Here's how the part is built. I have some questions about the finished solid (model axes, mm). A direction names the side the tool comes from. Coordinates: 2 decimals unless noted, no trailing zeros. Write each loop counter-clockwise with the first axis right and the second up, starting at its lowest first coordinate (ties: lowest second). Pieces come first, ordered by that corner, then holes.
```python
from build123d import *

# Parameters (mm, degrees)
SKETCH1_W           = 15
SKETCH1_H           = 100
BOSS_EXTRUDE1_DEPTH = 103
SKETCH2_W           = 15
SKETCH2_H           = 2
BOSS_EXTRUDE2_DEPTH = 15
SKETCH3_W           = 15
SKETCH3_H           = 2
BOSS_EXTRUDE3_DEPTH = 15
SKETCH4_R           = 2.15
CUT_EXTRUDE1_DEPTH  = 15
CHAMFER1_SIZE       = 1


with BuildPart() as part:
    # Sketch1 → Boss-Extrude1 (new body)
    with BuildSketch(Plane(origin=(0, 0, 0), x_dir=(1, 0, 0), z_dir=(0, 1, 0))):
        with Locations((7.5, 50)):
            Rectangle(SKETCH1_W, SKETCH1_H)
    extrude(amount=BOSS_EXTRUDE1_DEPTH)

    # Sketch2 → Boss-Extrude2 (add)
    with BuildSketch(Plane.ZY):
        with Locations((-50, 1)):
            Rectangle(SKETCH2_W, SKETCH2_H)
    extrude(amount=BOSS_EXTRUDE2_DEPTH)

    # Sketch3 → Boss-Extrude3 (add)
    with BuildSketch(Plane(origin=(15, 0, 0), x_dir=(0, 0, -1), z_dir=(1, 0, 0))):
        with Locations((50, 1)):
            Rectangle(SKETCH3_W, SKETCH3_H)
    extrude(amount=BOSS_EXTRUDE3_DEPTH)

    # Sketch4 → Cut-Extrude1 (cut)
    with BuildSketch(Plane(origin=(0, 2, 0), x_dir=(1, 0, 0), z_dir=(0, 1, 0))):
        with Locations(Location((-7.5, 50, 0), (0, 0, 270))):
            Circle(SKETCH4_R)
        with Locations(Location((22.5, 50, 0), (0, 0, 270))):
            Circle(SKETCH4_R)
    extrude(amount=-CUT_EXTRUDE1_DEPTH, mode=Mode.SUBTRACT)

    # Chamfer1
    chamfer1_edges = [part.edges().sort_by_distance(p)[0] for p in [
        (-7.5, 2, -52.15),
        (22.5, 2, -52.15),
    ]]
    chamfer(chamfer1_edges, length=CHAMFER1_SIZE)


solid = part.part
```
1) Imagine slicing it at B-B on x = -7.5. Please give me the cut outline in (y, z), then the cut area to 3 significant figures.
Values follow:
outline: (0, -57.5) - (2, -57.5) - (2, -53.15) - (1, -52.15) - (0, -52.15) - close; (0, -47.85) - (1, -47.85) - (2, -46.85) - (2, -42.5) - (0, -42.5) - close
area: 20.4 mm2
2) On a 3-axis mill with a long thin cutter (end or side, diameter ignored), from which of +Z, -Z, +X, -X, +Y, -Y can I reach the whole of each face in a straight line? I mean faces 1 (the face through (7, 103, -51)), 2 (the face through (-7.4, 2, -53.4)). Say none if no direction works.
Values follow:
face 1: +Z, -Z, +X, -X, +Y
face 2: +Z, -Z, -X, +Y
3) Imagine slicing it at C-C on y = 95. Please give me the cut outline in (x, z), then the cut area to 3 significant figures.
Values follow:
outline: (0, -100) - (15, -100) - (15, 0) - (0, 0) - close
area: 1,500 mm2
4) Imagine slicing it at D-D on z = -90. Please give me the cut outline in (x, y), then the cut area to 4 significant figures.
Values follow:
outline: (0, 0) - (15, 0) - (15, 103) - (0, 103) - close
area: 1,545 mm2
5) Will these pins go through, and if not, where does the flat tip stop? pin 1 (4 mm diameter, centred on x = 17.5, y = 74.5, fed in from +Z); pin 2 (5 mm diameter, centred on y = 15.5, z = -38.5, fed in from -X); pin 3 (2 mm diameter, centred on x = -9, y = 1, fed in from +Z); pin 4 (6 mm diameter, centred on y = 90, z = -29.5, fed in from +X).
Values follow:
pin 1: passes through
pin 2: stops at x = 0
pin 3: stops at z = -42.5
pin 4: stops at x = 15
6) I need wall thicknesses on probe 1 along X at (y, z) = (64.5, -76.5); probe 2 along Y at (x, z) = (-6, -57). Which ranges of each line are inside material? Lowest first, please.
Values follow:
probe 1: x = 0 to 15
probe 2: y = 0 to 2
7) We'd pull the mould along Z, two halves only. Please class faces 3 (the face through (-6.85, 0.51, -47.95)), 4 (the face through (7, 51, 0)), 5 (the face through (22.4, 2, -46.6)): pulls with the +Z half, pulls with the -Z half, needs draft (parallel to the pull), parting line crosses it, or undercut.
Values follow:
face 3: undercut
face 4: pulls with the +Z half
face 5: needs draft
8) Imagine slicing it at A-A on z = -50. Please give me the cut outline in (x, y).
Values follow:
outline: (-15, 0) - (-9.65, 0) - (-9.65, 1) - (-10.65, 2) - (-15, 2) - close; (-5.35, 0) - (20.35, 0) - (20.35, 1) - (19.35, 2) - (15, 2) - (15, 103) - (0, 103) - (0, 2) - (-4.35, 2) - (-5.35, 1) - close; (24.65, 0) - (30, 0) - (30, 2) - (25.65, 2) - (24.65, 1) - close
